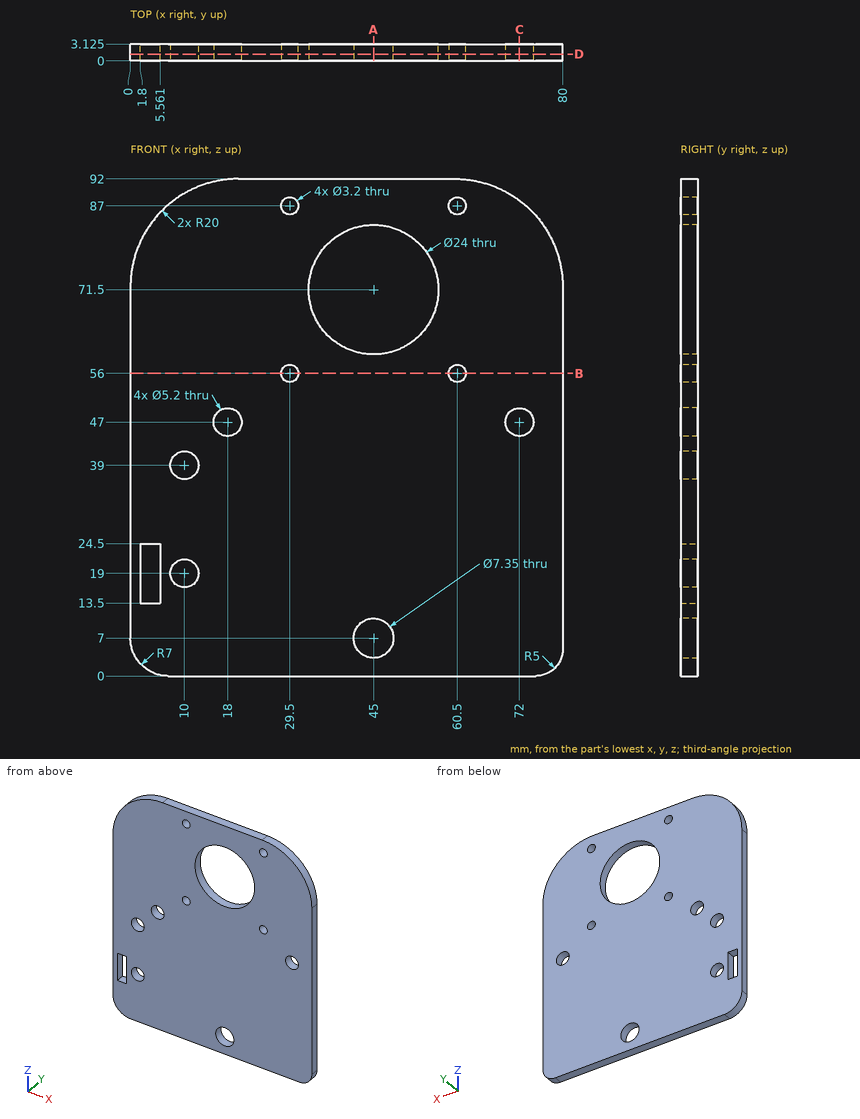
Source: three-view drawing plus pictorial views. Frame: mm from the lowest corner of the part. Give positions to 0.01 mm unless a question says otherwise; leave off trailing zeros. Write each loop counter-clockwise with the first axis right and the second up, starting at its lowest first coordinate (ties: lowest second). Pieces come first, ordered by that corner, then holes. Notation, with made-up numbers: (46.5, 77) -> (93.5, 77) arc R23 ccw to (93.5, 89) -> close; hole circle Ø7 at (-32, -22.75). An arc over 180 degrees is marked (long way). Answer in a Markdown table with one row per item.
(1) Section query B-B on z = 56. Return loops of the section in (x, y) (1 decimal).
Answers below:
| item | result |
|---|---|
| outline | (0, 0) -> (27.9, 0) -> (27.9, 3.1) -> (0, 3.1) -> close; (31.1, 0) -> (58.9, 0) -> (58.9, 3.1) -> (31.1, 3.1) -> close; (62.1, 0) -> (80, 0) -> (80, 3.1) -> (62.1, 3.1) -> close |
(2) Section query C-C on x = 72. Return loops of the section in (y, z) (1 decimal).
Answers below:
| item | result |
|---|---|
| outline | (0, 0) -> (3.1, 0) -> (3.1, 44.4) -> (0, 44.4) -> close; (0, 49.6) -> (3.1, 49.6) -> (3.1, 88) -> (0, 88) -> close |
(3) Section query A-A on x = 45. Return loops of the section in (y, z) (1 decimal).
Answers below:
| item | result |
|---|---|
| outline | (0, 0) -> (3.1, 0) -> (3.1, 3.3) -> (0, 3.3) -> close; (0, 10.7) -> (3.1, 10.7) -> (3.1, 59.5) -> (0, 59.5) -> close; (0, 83.5) -> (3.1, 83.5) -> (3.1, 92) -> (0, 92) -> close |
(4) Section query D-D on y = 1.25. State how many separate pieces and enclosed holes the cut face has, then the cut area to 3 significant figures.
Answers below:
| item | result |
|---|---|
| separate pieces | 1 |
| enclosed holes | 11 |
| area | 6,520 mm^2 |
(5) Pin query (flat end, axial travel): pin 1 (1.6 mm diameter, centred on x = 3.5, y = 1, fed in from -Z); pin 2 (6 mm diameter, centred on x = 72, z = 47, fed in from +Y) (3 decimals). Return the tip coordinate at first contact, or that it passes through.
Answers below:
| item | result |
|---|---|
| pin 1 | z = 0.54 |
| pin 2 | y = 3.125 |
(6) Ray query, line 1 along Z through (x, y) = (45, 1.8) (1 decimal); line 2 along X through (y, z) = (1.6, 56); line 3 along Z through (x, y) = (29.5, 2.2). Return the intervals inside material, ascending. Write a range as [from, to].
Answers below:
| item | result |
|---|---|
| line 1 | [0, 3.3], [10.7, 59.5], [83.5, 92] |
| line 2 | [0, 27.9], [31.1, 58.9], [62.1, 80] |
| line 3 | [0, 54.4], [57.6, 85.4], [88.6, 92] |
